Here's how the part is built. I have some questions about the finished solid (model axes, mm). A direction names the side the tool comes from. Coordinates: 2 decimals unless noted, no trailing zeros. Write each loop counter-clockwise with the first axis right and the second up, starting at its lowest first coordinate (ties: lowest second). Pieces come first, ordered by that corner, then holes.
(1) For pin 1 Ø1.5 at (y, z) = (-6, -1) entering from +X; pin 2 Ø5 at (x, y) = (-26, 6.5) entering from +Z, each with a flat end and sliding along its axis, tell me the tip position at first contact or that it passes through.
(2) Which directions (+Z, -Z, +X, -X, +Y, -Y) give clear straight access to the entire face, cutting with the end or side of a thin tool? Please do faces 1 (the flat face through (-23.293, 0.052, -0.018)), 2 (the cylindrical face through (-32.34, -1.33, 0.49)).
(3) Imagine slicing it at A-A, the plane z = 0. List the corners of the cut face in (x, y) for me.
(4) Imagine slicing it at B-B, the plane y = -14.5. List the corners of the cut face in (x, z) for me, plus the area to 3 significant figures.
(5) Imagine slicing it at C-C, the plane y = 1.5. State how many separate pieces and enclosed holes the cut face has, plus the area to 3 significant figures.
(6) Thinking about a two-plate mould opening in Y: for faces 3 (the cylindrical face through (-19.84, -39.085, -0.381)), 4 (the cylindrical face through (-19.58, 37.26, 0.49)), 5 (the flat face through (0, 0, 0)), 6 (the cylindrical face through (-0.17, 15.08, -1.26)), which applies, released by +Y, released by -Y, zero draft, split by the parting line, or undercut?
(7) Please list where these lines run through material, in increasing order: probe 1 along X at (y, z) = (12, -1.1); probe 2 along X at (y, z) = (31, 0.25); probe 3 along Y at (x, z) = (-14, 0.85).
```python
from build123d import *

# Parameters (mm, degrees)
F0_R = 1.27


with BuildPart() as f2:
    # F2: sweep along a path in F1
    with BuildLine(Plane.XY) as f2_path:
        Line((0, 0), (0, 29.7363953829))
        ThreePointArc((0, 29.7363953829), (-1.8598719395, 34.2265234434), (-6.35, 36.0863953829))
        Line((-6.35, 36.0863953829), (-31.1682708561, 36.0863953829))
        Line((-31.1682708561, 36.0863953829), (-31.1682708561, -37.6992039382))
        Line((-31.1682708561, -37.6992039382), (-8.8609969243, -38.042396307))
        Line((-8.8609969243, -38.042396307), (-8.8609969243, 20.9860876203))
        Line((-8.8609969243, 20.9860876203), (-22.2453605384, 22.7020308375))
        Line((-22.2453605384, 22.7020308375), (-23.2749264687, 0.0515673637))
    # F0 (on Front) → F2 (sweep)
    with BuildSketch(Plane.XZ):
        Circle(F0_R)
    sweep(path=f2_path.line, transition=Transition.RIGHT)


solid = f2.part
```
Recorded:
1. pin 1: stops at x = -7.62
1. pin 2: stops at z = 1.16
2. face 1: +Z, -Z
2. face 2: none
3. outline: (-32.44, -38.95) - (-7.59, -39.33) - (-7.59, 22.1) - (-23.45, 24.14) - (-24.54, 0.11) - (-22.01, -0.01) - (-21.04, 21.27) - (-10.13, 19.87) - (-10.13, -36.75) - (-29.9, -36.45) - (-29.9, 34.82) - (-6.35, 34.82) arc R5.08 cw to (-1.27, 29.74) - (-1.27, 0) - (1.27, 0) - (1.27, 29.74) arc R7.62 ccw to (-6.35, 37.36) - (-32.44, 37.36) - close
4. outline: circle Ø2.54 at (-31.17, 0); circle Ø2.54 at (-8.86, 0)
4. area: 10.1 mm2
5. separate pieces: 4
5. enclosed holes: 0
5. area: 20.3 mm2
6. face 3: undercut
6. face 4: undercut
6. face 5: released by -Y
6. face 6: zero draft
7. probe 1: x = -31.8 to -30.53, -23.37 to -22.1, -9.5 to -8.23, -0.63 to 0.63
7. probe 2: x = -32.41 to -29.92, -1.4 to 1.14
7. probe 3: y = -38.91 to -37.02, 20.69 to 22.6, 35.14 to 37.03
